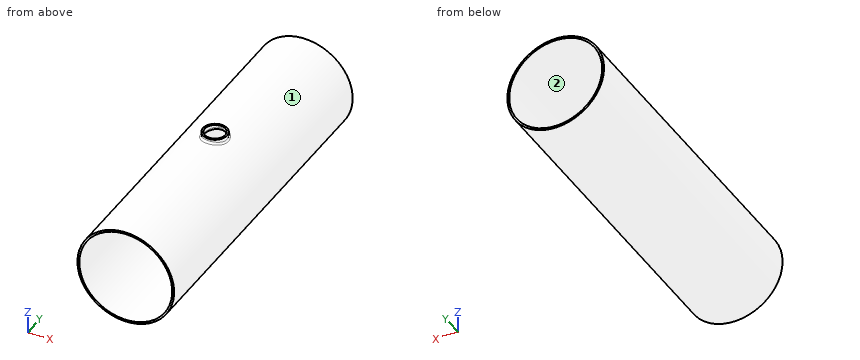
Autodesk Inventor part; units mm, degrees
ref_plane "YZ Plane" through (0, 0, 0) normal (1, 0, 0) x (0, 1, 0)
ref_plane "XZ Plane" through (0, 0, 0) normal (0, 1, 0) x (-1, 0, 0)
ref_plane "XY Plane" through (0, 0, 0) normal (0, 0, 1) x (1, 0, 0)
sketch "Szkic8" plane through (0, 0, 0) normal (0, 1, 0) x (-1, 0, 0)
  circle A0 centre (0, 0) radius 50.8
  circle A1 centre (0, 0) radius 48.8
  dimension "d53" = 101.6
  dimension "d54" = 2
extrude "Wyciągnięcie proste2" add sketch "Szkic8" along normal mid plane 348
sketch "Szkic13" plane through (0, 0, 0) normal (0, 0, 1) x (1, 0, 0)
  circle A0 centre (0, 0) radius 12.7
  circle A1 centre (0, 0) radius 10.7
  dimension "d67" = 25.4
  dimension "d68" = 2
extrude "Wyciągnięcie proste6" add sketch "Szkic13" along normal blind 55
sketch "Szkic14" plane through (0, 0, 55) normal (0, 0, 1) x (1, 0, 0)
  circle A0 centre (0, 0) radius 10.7
extrude "Wyciągnięcie proste7" cut sketch "Szkic14" against normal blind 55
sketch "Szkic15" plane through (0, -174, 0) normal (0, -1, 0) x (1, 0, 0)
  circle A0 centre (0, 0) radius 48.8
extrude "Wyciągnięcie proste8" cut sketch "Szkic15" against normal blind 348
fillet "Zaokrąglenie3" radius 2 2 edges at (0, 12.7, 50.8) (-0.0026, -12.7, 50.8)
fillet "Zaokrąglenie4" radius 4 2 edges at (0.0357, -10.6999, 48.8) (-0.0345, 10.6999, 48.8)
equation "\"d53\" = OD"
equation "\"d54\" = THK"
equation "\"d55\" = L1"
equation "\"d67\" = OD2"
equation "\"d68\" = THK"
equation "\"d69\" = L2"
equation "\"d71\" = L2"
equation "\"d73\" = L1"
equation "\"d75\" = THK"
equation "\"d76\" = 2 * THK"
equation "\"SzerokośćGięciaPodcięcia\" = Grubość"
equation "\"RozmiarPodcięciaNarożnika\" = 4 * Grubość"
equation "\"PromieńPrzejścia\" = PromieńGięcia"
equation "\"Rozmiar_promienia_Jacobiego\" = PromieńGięcia"
equation "\"Wielk_odstępu\" = Grubość"
equation "\"d2\" = PromieńGięcia"
equation "\"d23\" = PromieńGięcia"
equation "\"OD\" = 101.6"
equation "\"THK\" = 2"
equation "\"L1\" = 348"
equation "\"L2\" = 55"
equation "\"OD2\" = 25.4"
properties part number "Trójnik red. krótki  Ø101,6 25,4 101,6 s=2 L=348" material "304"
Could you check a few things on this model? Use its own coordinates, in mm. Face numbers are marked on the shaded views. Round coordinates to 2 decimals unless told otherwise and drop trailing zeros. Loops run counter-clockwise (first coordinate to the right, second up) from the corner with the lowest first, then second, coordinate; pieces in that order, holes last. Notation, with made-up numbers: (78, 25.5) -> (93, 25.5) arc R26 ccw to (93, 63.5) -> close; hole circle Ø1 at (64.25, 32.5). An arc over 180 degrees is marked (long way). Put each result on its own line as item: value.
Q1. I want a section at A-A on z = 0. Write out the boundary of the cut face in (x, y).
Checks:
outline: (-50.8, -174) -> (-48.8, -174) -> (-48.8, 174) -> (-50.8, 174) -> close; (48.8, -174) -> (50.8, -174) -> (50.8, 174) -> (48.8, 174) -> close
Q2. I want a section at D-D on x = 0. Give the number of separate pieces and of enclosed holes in the cut face, and give its area (3 significant figures).
Checks:
separate pieces: 3
enclosed holes: 0
area: 1,360 mm2
Q3. I want a section at B-B on x = 44. Write out the boundary of the cut face in (y, z), and give its area (3 significant figures).
Checks:
outline: (-174, -25.39) -> (174, -25.39) -> (174, -21.11) -> (-174, -21.11) -> close; (-174, 21.11) -> (174, 21.11) -> (174, 25.39) -> (-174, 25.39) -> close
area: 2,980 mm2
Q4. I want a section at C-C on y = -132.5. Write out the boundary of the cut face in (x, z).
Checks:
outline: circle Ø101.6 at (0, 0); hole circle Ø97.6 at (0, 0)
Q5. Please list where these lines run through material, in increasing order: line 1 (Y direction, x = 0, z = 54); line 2 (Z direction, x = 0.5, y = -121). Write a range as from..to.
Checks:
line 1: -12.7..-10.7, 10.7..12.7
line 2: -50.8..-48.8, 48.8..50.8
Q6. For pin 1 Ø3 at (x, y) = (2.5, -91) entering from +Z; pin 2 Ø10 at (x, y) = (-19.5, -102.5) entering from -Z; pin 3 Ø8 at (y, z) = (37, 24.5) entering from +X; pin 4 Ø12 at (x, z) = (26.5, 35.5) entering from +Y, each with a flat end and sliding along its axis, tell me the tip position at first contact or that it passes through.
Checks:
pin 1: z = 50.79
pin 2: z = -48.69
pin 3: x = 46.48
pin 4: y = 174
Q7. Thinking about a two-plate mould opening in Z: for the marked faces 1 and 2, which applies, pulls with the +Z half, pulls with the -Z half, needs draft (parallel to the pull), parting line crosses it, or undercut?
Checks:
face 1: parting line crosses it
face 2: undercut
